from build123d import *

# Parameters (mm, degrees)
SKETCH1_W           = 127
SKETCH1_H           = 127
BOSS_EXTRUDE1_DEPTH = 107.95
SKETCH2_W           = 88.9
SKETCH2_H           = 88.9
CUT_EXTRUDE1_DEPTH  = 179.366063196
SKETCH4_W           = 88.9
SKETCH4_H           = 88.9
CUT_EXTRUDE4_DEPTH  = 179.366063196
CUT_EXTRUDE5_REACH  = 142.42
SKETCH6_W           = 38.1
SKETCH6_H           = 38.1
FILLET1_R           = 10
CHAMFER2_SIZE       = 12.7
SKETCH7_W           = 25.4
SKETCH7_H           = 25.4
SKETCH7_R           = 6.35
BOSS_EXTRUDE2_DEPTH = 12.7
FILLET2_START       = 19.05
FILLET2_DEPTH       = 101.6


with BuildPart() as part:
    # Sketch1 → Boss-Extrude1 (new body)
    with BuildSketch(Plane(origin=(0, 0, 0), x_dir=(1, 0, 0), z_dir=(0, 1, 0))):
        Rectangle(SKETCH1_W, SKETCH1_H)
    extrude(amount=BOSS_EXTRUDE1_DEPTH)

    # Sketch2 → Cut-Extrude1 (cut, through all)
    with BuildSketch(Plane.XY.offset(63.5)):
        with Locations((0, 63.5)):
            Rectangle(SKETCH2_W, SKETCH2_H)
    extrude(amount=-CUT_EXTRUDE1_DEPTH, mode=Mode.SUBTRACT)

    # Sketch4 → Cut-Extrude4 (cut, through all)
    with BuildSketch(Plane(origin=(63.5, 0, 0), x_dir=(0, 0, -1), z_dir=(1, 0, 0))):
        with Locations((0, 63.5)):
            Rectangle(SKETCH4_W, SKETCH4_H)
    extrude(amount=-CUT_EXTRUDE4_DEPTH, mode=Mode.SUBTRACT)

    # Sketch6 → Cut-Extrude5 (cut, up to next)
    with BuildSketch(Plane.XZ, mode=Mode.PRIVATE) as cut_extrude5_sk1:
        Rectangle(SKETCH6_W, SKETCH6_H)
    cut_extrude5_tool1 = extrude(cut_extrude5_sk1.sketch, amount=-CUT_EXTRUDE5_REACH, mode=Mode.PRIVATE) & part.part
    add(cut_extrude5_tool1.solids().sort_by_distance((0, 0, 0))[0], mode=Mode.SUBTRACT)

    # Fillet1
    fillet1_edges = [part.edges().sort_by_distance(p)[0] for p in [
        (63.5, 0, 0),
        (0, 0, -63.5),
        (-63.5, 0, 0),
        (0, 0, 63.5),
        (63.5, 53.975, 63.5),
        (63.5, 53.975, -63.5),
        (-63.5, 53.975, -63.5),
        (-63.5, 53.975, 63.5),
    ]]
    fillet(fillet1_edges, radius=FILLET1_R)

    # Chamfer2
    chamfer2_edges = [part.edges().sort_by_distance(p)[0] for p in [
        (-44.45, 63.5, -44.45),
        (44.45, 63.5, -44.45),
        (-44.45, 63.5, 44.45),
        (44.45, 63.5, 44.45),
    ]]
    chamfer(chamfer2_edges, length=CHAMFER2_SIZE)

    # Sketch7 → Boss-Extrude2 (add)
    # profile 1 of 4: a face of its own
    with BuildSketch(Plane(origin=(0, 107.95, 0), x_dir=(1, 0, 0), z_dir=(0, 1, 0))):
        with Locations((50.8, 50.8)):
            Rectangle(SKETCH7_W, SKETCH7_H)
        with Locations(Location((50.8, 50.8, 0), (0, 0, 90))):
            Circle(SKETCH7_R, mode=Mode.SUBTRACT)
    # profile 2 of 4: a face of its own
    with BuildSketch(Plane(origin=(0, 107.95, 0), x_dir=(1, 0, 0), z_dir=(0, 1, 0))):
        with Locations((-50.8, 50.8)):
            Rectangle(SKETCH7_W, SKETCH7_H)
        with Locations(Location((-50.8, 50.8, 0), (0, 0, 45))):
            Circle(SKETCH7_R, mode=Mode.SUBTRACT)
    # profile 3 of 4: a face of its own
    with BuildSketch(Plane(origin=(0, 107.95, 0), x_dir=(1, 0, 0), z_dir=(0, 1, 0))):
        with Locations((-50.8, -50.8)):
            Rectangle(SKETCH7_W, SKETCH7_H)
        with Locations(Location((-50.8, -50.8, 0), (0, 0, 90))):
            Circle(SKETCH7_R, mode=Mode.SUBTRACT)
    # profile 4 of 4: a face of its own
    with BuildSketch(Plane(origin=(0, 107.95, 0), x_dir=(1, 0, 0), z_dir=(0, 1, 0))):
        with Locations((50.8, -50.8)):
            Rectangle(SKETCH7_W, SKETCH7_H)
        with Locations(Location((50.8, -50.8, 0), (0, 0, 45))):
            Circle(SKETCH7_R, mode=Mode.SUBTRACT)
    extrude(amount=BOSS_EXTRUDE2_DEPTH)

    # Fillet2: read off the stored shape, not the designer's step
    # Fillet2 outline → Fillet2 (cut)
    with BuildSketch(Plane(origin=(0, 0, 0), x_dir=(1, 0, 0), z_dir=(0, 1, 0)).offset(FILLET2_START)):
        with BuildLine():
            Line((63.5, -63.5), (63.5, -53.5))
            ThreePointArc((63.5, -53.5), (60.571067812, -60.571067812), (53.5, -63.5))
            Line((53.5, -63.5), (63.5, -63.5))
        make_face()
        with BuildLine():
            Line((63.5, -48.1), (63.5, -38.1))
            Line((63.5, -38.1), (53.5, -38.1))
            ThreePointArc((53.5, -38.1), (60.571067812, -41.028932188), (63.5, -48.1))
        make_face()
        with BuildLine():
            ThreePointArc((48.1, -63.5), (41.028932188, -60.571067812), (38.1, -53.5))
            Line((38.1, -53.5), (38.1, -63.5))
            Line((38.1, -63.5), (48.1, -63.5))
        make_face()
        with BuildLine():
            ThreePointArc((38.1, -48.1), (41.028932188, -41.028932188), (48.1, -38.1))
            Line((48.1, -38.1), (38.1, -38.1))
            Line((38.1, -38.1), (38.1, -48.1))
        make_face()
        with BuildLine():
            Line((53.5, 38.1), (63.5, 38.1))
            Line((63.5, 38.1), (63.5, 48.1))
            ThreePointArc((63.5, 48.1), (60.571067812, 41.028932188), (53.5, 38.1))
        make_face()
        with BuildLine():
            Line((-38.1, -63.5), (-38.1, -53.5))
            ThreePointArc((-38.1, -53.5), (-41.028932188, -60.571067812), (-48.1, -63.5))
            Line((-48.1, -63.5), (-38.1, -63.5))
        make_face()
        with BuildLine():
            Line((38.1, 38.1), (48.1, 38.1))
            ThreePointArc((48.1, 38.1), (41.028932188, 41.028932188), (38.1, 48.1))
            Line((38.1, 48.1), (38.1, 38.1))
        make_face()
        with BuildLine():
            ThreePointArc((-48.1, -38.1), (-41.028932188, -41.028932188), (-38.1, -48.1))
            Line((-38.1, -48.1), (-38.1, -38.1))
            Line((-38.1, -38.1), (-48.1, -38.1))
        make_face()
        with BuildLine():
            ThreePointArc((53.5, 63.5), (60.571067812, 60.571067812), (63.5, 53.5))
            Line((63.5, 53.5), (63.5, 63.5))
            Line((63.5, 63.5), (53.5, 63.5))
        make_face()
        with BuildLine():
            Line((-63.5, -63.5), (-53.5, -63.5))
            ThreePointArc((-53.5, -63.5), (-60.571067812, -60.571067812), (-63.5, -53.5))
            Line((-63.5, -53.5), (-63.5, -63.5))
        make_face()
        with BuildLine():
            Line((38.1, 63.5), (38.1, 53.5))
            ThreePointArc((38.1, 53.5), (41.028932188, 60.571067812), (48.1, 63.5))
            Line((48.1, 63.5), (38.1, 63.5))
        make_face()
        with BuildLine():
            Line((-53.5, -38.1), (-63.5, -38.1))
            Line((-63.5, -38.1), (-63.5, -48.1))
            ThreePointArc((-63.5, -48.1), (-60.571067812, -41.028932188), (-53.5, -38.1))
        make_face()
        with BuildLine():
            Line((-38.1, 53.5), (-38.1, 63.5))
            Line((-38.1, 63.5), (-48.1, 63.5))
            ThreePointArc((-48.1, 63.5), (-41.028932188, 60.571067812), (-38.1, 53.5))
        make_face()
        with BuildLine():
            Line((-63.5, 38.1), (-53.5, 38.1))
            ThreePointArc((-53.5, 38.1), (-60.571067812, 41.028932188), (-63.5, 48.1))
            Line((-63.5, 48.1), (-63.5, 38.1))
        make_face()
        with BuildLine():
            Line((-38.1, 38.1), (-38.1, 48.1))
            ThreePointArc((-38.1, 48.1), (-41.028932188, 41.028932188), (-48.1, 38.1))
            Line((-48.1, 38.1), (-38.1, 38.1))
        make_face()
        with BuildLine():
            ThreePointArc((-63.5, 53.5), (-60.571067812, 60.571067812), (-53.5, 63.5))
            Line((-53.5, 63.5), (-63.5, 63.5))
            Line((-63.5, 63.5), (-63.5, 53.5))
        make_face()
    extrude(amount=FILLET2_DEPTH, mode=Mode.SUBTRACT)


solid = part.part
CAD build for the part. Positions are in the model's coordinates, mm. A direction names the side the tool comes from. Round coordinates to 2 decimals unless told otherwise and drop trailing zeros. Write each loop counter-clockwise with the first axis right and the second up, starting at its lowest first coordinate (ties: lowest second). Pieces come first, ordered by that corner, then holes. Notation, with made-up numbers: (-11, -21) -> (25, -21) arc R19 cw to (25, 6) -> close; hole circle Ø11 at (-11, 7.5). An arc over 180 degrees is marked (long way). Answer as a JSON object with one key per item and string values.
(1) Band-saw the part on A-A, the plane z = -2.5. List the corners of the cut face in (x, y), then the cut area to 3 significant figures.
Reported:
{"outline": "(-63.5, 10) arc R10 ccw to (-53.5, 0) -> (-19.05, 0) -> (-19.05, 19.05) -> (-63.5, 19.05) -> close; (19.05, 0) -> (53.5, 0) arc R10 ccw to (63.5, 10) -> (63.5, 19.05) -> (19.05, 19.05) -> close", "area": "1,650 mm^2"}
(2) Band-saw the part on C-C, the plane y = 58. Count the separate pieces of the cut face and the enclosed holes in it, then the cut area to 3 significant figures.
Reported:
{"separate pieces": "4", "enclosed holes": "0", "area": "1,040 mm^2"}
(3) Band-saw the part on D-D, the plane z = 50.8. List the corners of the cut face in (x, y).
Reported:
{"outline": "(-63.5, 10) arc R10 ccw to (-53.5, 0) -> (53.5, 0) arc R10 ccw to (63.5, 10) -> (63.5, 120.65) -> (57.15, 120.65) -> (57.15, 107.95) -> (50.8, 107.95) -> (50.8, 19.05) -> (-50.8, 19.05) -> (-50.8, 107.95) -> (-57.15, 107.95) -> (-57.15, 120.65) -> (-63.5, 120.65) -> close; (-44.45, 107.95) -> (-38.1, 107.95) -> (-38.1, 120.65) -> (-44.45, 120.65) -> close; (38.1, 107.95) -> (44.45, 107.95) -> (44.45, 120.65) -> (38.1, 120.65) -> close"}
(4) Probe probe 1 along X at (y, z) = (118, 50.8); probe 2 along Y at (x, z) = (-47, 40). List the from-to ranges inside material, lowest first. Write a range as [from, to].
Reported:
{"probe 1": "x = [-63.5, -57.15], [-44.45, -38.1], [38.1, 44.45], [57.15, 63.5]", "probe 2": "y = [0, 19.05], [107.95, 120.65]"}
(5) Which spindle directions (+Z, -Z, +X, -X, +Y, -Y) get a long thin tool onto all of the face, cutting with end or side? Do faces 4 (the face through (53, 107.95, 53)), 5 (the face through (-51, 114, -38.1)), 6 (the face through (-44.45, 63, 60)). Say none if no direction does.
Reported:
{"face 4": "+Y", "face 5": "+X, -X, +Y", "face 6": "+Z, -Z"}
(6) Pin check, flat tips, straight feed: P1, Ø6, axis at x = 60.5, y = 59, coming from the +Z side; P2, Ø1, axis at x = -7.5, z = 49, coming from the +Y side; P3, Ø4.5, axis at y = 63, z = 60.5, coming from the -X side. Stop position of each tip, or through.
Reported:
{"P1": "stops at z = 62.67", "P2": "stops at y = 19.05", "P3": "stops at x = -62.3"}
(7) Band-saw the part on B-B, the plane x = -50.8. List the corners of the cut face in (y, z), then the cut area to 3 significant figures.
Reported:
{"outline": "(0, -53.5) arc R10 ccw to (10, -63.5) -> (120.65, -63.5) -> (120.65, -57.15) -> (107.95, -57.15) -> (107.95, -50.8) -> (19.05, -50.8) -> (19.05, 50.8) -> (107.95, 50.8) -> (107.95, 57.15) -> (120.65, 57.15) -> (120.65, 63.5) -> (10, 63.5) arc R10 ccw to (0, 53.5) -> close; (107.95, -44.45) -> (120.65, -44.45) -> (120.65, -38.1) -> (107.95, -38.1) -> close; (107.95, 38.1) -> (120.65, 38.1) -> (120.65, 44.45) -> (107.95, 44.45) -> close", "area": "4,960 mm^2"}
(8) Two-plate mould, pull along Z, no slides. Class faces 1 (the face through (47.8, 120.65, 45)), 2 (the face through (0.75, 2.85, -60.49)), 3 (the face through (-53, 107.95, -53)): +Z half, -Z half, draft (parallel to the pull), parting line (faces both ways), or undercut.
Reported:
{"face 1": "draft", "face 2": "-Z half", "face 3": "undercut"}
